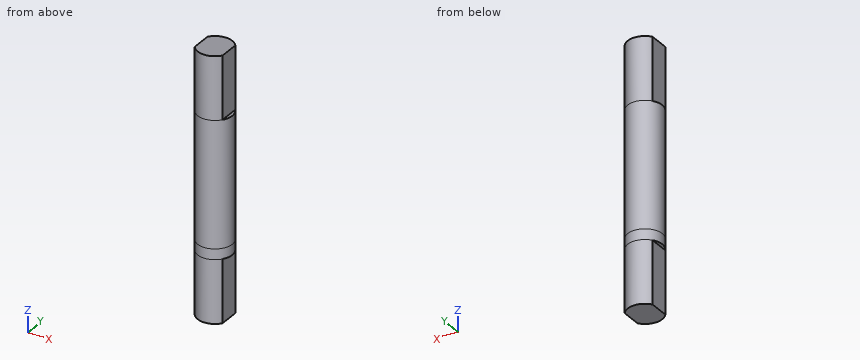
from build123d import *

# Parameters (mm, degrees)
SKETCH1_R                = 2.48
BOSS_EXTRUDE1_DEPTH      = 11
BOSS_EXTRUDE1_DEPTH_BACK = 5
SKETCH2_R                = 2.48
BOSS_EXTRUDE2_DEPTH      = 2
BOSS_EXTRUDE3_DEPTH      = 9
SKETCH4_R                = 2.48
BOSS_EXTRUDE4_DEPTH      = 1.5
BOSS_EXTRUDE5_DEPTH      = 9


with BuildPart() as part:
    # Sketch1 → Boss-Extrude1 (new body, two sides)
    with BuildSketch(Plane.XY) as boss_extrude1_sk:
        Circle(SKETCH1_R)
    extrude(amount=BOSS_EXTRUDE1_DEPTH)
    extrude(boss_extrude1_sk.sketch, amount=-BOSS_EXTRUDE1_DEPTH_BACK)

    # Sketch2 → Boss-Extrude2 (add)
    with BuildSketch(Plane.XY.offset(11)):
        Circle(SKETCH2_R)
    extrude(amount=BOSS_EXTRUDE2_DEPTH)

    # Sketch3 → Boss-Extrude3 (add)
    with BuildSketch(Plane.XY.offset(13)):
        with BuildLine():
            ThreePointArc((2, 1.466424222), (0, 2.48), (-2, 1.466424222))
            Line((-2, 1.466424222), (-2, -1.466424222))
            ThreePointArc((-2, -1.466424222), (0, -2.48), (2, -1.466424222))
            Line((2, -1.466424222), (2, 1.466424222))
        make_face()
    extrude(amount=BOSS_EXTRUDE3_DEPTH)

    # Sketch4 → Boss-Extrude4 (add)
    with BuildSketch(Plane(origin=(0, 0, -5), x_dir=(-1, 0, 0), z_dir=(0, 0, -1))):
        Circle(SKETCH4_R)
    extrude(amount=BOSS_EXTRUDE4_DEPTH)

    # Sketch5 → Boss-Extrude5 (add)
    with BuildSketch(Plane(origin=(0, 0, -6.5), x_dir=(-1, 0, 0), z_dir=(0, 0, -1))):
        with BuildLine():
            ThreePointArc((2, 1.466424222), (0, 2.48), (-2, 1.466424222))
            Line((-2, 1.466424222), (-2, -1.466424222))
            ThreePointArc((-2, -1.466424222), (0, -2.48), (2, -1.466424222))
            Line((2, -1.466424222), (2, 1.466424222))
        make_face()
    extrude(amount=BOSS_EXTRUDE5_DEPTH)


solid = part.part
Geometry: final body of the model. Coordinates: model frame, mm. Coordinates: 2 decimals unless noted, no trailing zeros. Loops run counter-clockwise (first coordinate to the right, second up) from the corner with the lowest first, then second, coordinate; pieces in that order, holes last. Notation, with made-up numbers: M -7,52 L 49,52 A28 cw 49,78 Z; hole C -0.75,60.5 d6. An arc over 180 degrees is marked long. One line per item, written item: value. Start each with the question number.
1) Cut plane C-C (z = 9.5). Return loops of the section in (x, y), then the cut area to 3 significant figures.
2) Cut plane D-D (y = -1.9). Return loops of the section in (x, z), then the cut area to 3 significant figures.
3) Cut plane A-A (y = 0). Return loops of the section in (x, z).
4) Pin query (flat end, axial travel): P1, Ø0.9, axis at y = 0, z = 16.5, coming from the +X side; P2, Ø2.5, axis at y = -0.5, z = -10.5, coming from the -X side; P3, Ø1.5, axis at y = -0.5, z = -5, coming from the -X side; P4, Ø0.5, axis at x = 2.5, y = 0, coming from the -Z side. Return the tip coordinate at first contact, or that it passes through.
5) Material intervals for L1, parallel to Y at x = -0.1, z = 20; L2, parallel to X at y = -1, z = -7; L3, parallel to Z at x = 2.3, y = -0.5, sorted ascending. Write a range as from..to.
6) Cut plane B-B (x = -0.85). Return loops of the section in (y, z), then the cut area to 3 significant figures.
Evaluation:
1. outline: C 0,0 d4.96
1. area: 19.3 mm^2
2. outline: M -1.59,-15.5 L 1.59,-15.5 L 1.59,22 L -1.59,22 Z
2. area: 120 mm^2
3. outline: M -2.48,-6.5 L -2,-6.5 L -2,-15.5 L 2,-15.5 L 2,-6.5 L 2.48,-6.5 L 2.48,13 L 2,13 L 2,22 L -2,22 L -2,13 L -2.48,13 Z
4. P1: x = 2
4. P2: x = -2
4. P3: x = -2.48
4. P4: z = -6.5
5. L1: -2.48..2.48
5. L2: -2..2
5. L3: -6.5..13
6. outline: M -2.33,-15.5 L 2.33,-15.5 L 2.33,22 L -2.33,22 Z
6. area: 175 mm^2
